The listing builds one solid part. Answer for the finished solid, in the listing's coordinates (mm). A direction names the side the tool comes from. Give positions to 0.01 mm unless a question says otherwise; leave off trailing zeros. Order: outer loops, then holes, each group sorted by start corner. A loop starts at its lowest first (then second) coordinate and runs counter-clockwise, first axis right, second up. Notation, with made-up numbers: (42, -16.5) -> (64, -16.5) arc R21 cw to (64, 0.5) -> close; hole circle Ø6 at (-19, -37.75). An arc over 180 degrees is marked (long way). Answer as a JSON object with one key per item and string values. Group by question number.
```python
from build123d import *

# Parameters (mm, degrees)
F0_W     = 1.2
F0_H     = 0.3
F1_DEPTH = 4.7
F3_DEPTH = 1.05
F6_DEPTH = 2
F7_SIZE  = 1
F8_W     = 2.05
F8_H     = 0.3
F9_DEPTH = 125


with BuildPart() as f1:
    # F0 (on Front) → F1 (new body)
    with BuildSketch(Plane.XZ):
        with BuildLine():
            Line((0, 31.15), (0, 0))
            Line((0, 0), (19.75, 0))
            Line((19.75, 0), (19.75, 31.15))
            Line((19.75, 31.15), (18.55, 31.15))
            Line((18.55, 31.15), (10.275, 31.15))
            Line((10.275, 31.15), (10.275, 31.45))
            Line((10.275, 31.45), (18.55, 31.45))
            Line((18.55, 31.45), (19.75, 31.45))
            Line((19.75, 31.45), (19.75, 52.5))
            Line((19.75, 52.5), (19.75, 55.1716775767))
            ThreePointArc((19.75, 55.1716775767), (18.375, 59.5), (19.75, 63.8283224233))
            Line((19.75, 63.8283224233), (19.75, 65))
            Line((19.75, 65), (0, 65))
            Line((0, 65), (0, 63.8283224233))
            ThreePointArc((0, 63.8283224233), (1.0229892277, 61.7707377656), (1.375, 59.5))
            ThreePointArc((1.375, 59.5), (1.0229892277, 57.2292622344), (0, 55.1716775767))
            Line((0, 55.1716775767), (0, 52.5))
            Line((0, 52.5), (0, 31.45))
            Line((0, 31.45), (1.2, 31.45))
            Line((1.2, 31.45), (9.475, 31.45))
            Line((9.475, 31.45), (9.475, 31.15))
            Line((9.475, 31.15), (1.2, 31.15))
            Line((1.2, 31.15), (0, 31.15))
        make_face()
        with BuildLine():
            Line((-2, 52.5), (0, 52.5))
            Line((0, 52.5), (0, 55.1716775767))
            ThreePointArc((0, 55.1716775767), (-0.9094386331, 54.1103878035), (-2, 53.2362650918))
            Line((-2, 53.2362650918), (-2, 52.5))
        make_face()
        with BuildLine():
            Line((19.75, 55.1716775767), (19.75, 52.5))
            Line((19.75, 52.5), (21.75, 52.5))
            Line((21.75, 52.5), (21.75, 53.2362650918))
            ThreePointArc((21.75, 53.2362650918), (20.6594386331, 54.1103878035), (19.75, 55.1716775767))
        make_face()
        with Locations((0.6, 31.3)):
            Rectangle(F0_W, F0_H)
        with Locations((19.15, 31.3)):
            Rectangle(F0_W, F0_H)
    extrude(amount=F1_DEPTH)

    # F2 (on face) → F3 (cut)
    with BuildSketch(Plane.XZ.offset(4.7)):
        Polygon((13.475, 37.5), (6.275, 37.5), (6.275, 2.2), (6.275, 0), (13.475, 0), (13.475, 2.2), align=None)
    extrude(amount=-F3_DEPTH, mode=Mode.SUBTRACT)

    # F5 (on face) → F6 (join)
    with BuildSketch(Plane.XZ.offset(4.7)):
        with BuildLine():
            Line((-2, 52.5), (0, 52.5))
            Line((0, 52.5), (19.75, 52.5))
            Line((19.75, 52.5), (21.75, 52.5))
            Line((21.75, 52.5), (21.75, 53.2362650918))
            ThreePointArc((21.75, 53.2362650918), (18.5052276407, 58.1084342015), (19.75, 63.8283224233))
            Line((19.75, 63.8283224233), (19.75, 65))
            Line((19.75, 65), (0, 65))
            Line((0, 65), (0, 63.8283224233))
            ThreePointArc((0, 63.8283224233), (1.2447723593, 58.1084342015), (-2, 53.2362650918))
            Line((-2, 53.2362650918), (-2, 52.5))
        make_face()
    extrude(amount=F6_DEPTH)

    # F7
    f7_edges = [f1.edges().sort_by_distance(p)[0] for p in [
        (0, -2.35, 0),
        (19.75, -2.35, 0),
        (3.1375, -4.7, 0),
        (16.6125, -4.7, 0),
        (9.875, -3.65, 0),
    ]]
    chamfer(f7_edges, length=F7_SIZE)

    # F8 (on face) → F9 (cut, symmetric)
    with BuildSketch(Plane(origin=(9.475, 0, 0), x_dir=(0, -1, 0), z_dir=(-1, 0, 0))):
        with Locations((1.825, 31.3)):
            Rectangle(F8_W, F8_H)
    extrude(amount=F9_DEPTH, both=True, mode=Mode.SUBTRACT)


solid = f1.part
```
(1) A cutting plane is placed at B-B (y = -2). Determine the outline of the cut face in (x, z) (3 decimals), and give its area (3 significant figures).
(2) Find the intervals of material crossed by line 1 along Z through (x, y) = (11.75, -0.75); line 2 along X through (y, z) = (-4.5, 5.5) (3 decimals); line 3 along Y through (x, z) = (14.25, 6), in increasing order. Write a range as [from, to].
(3) Flat-ended cylindrical pins translate along their axes: pin 1 Ø8 at (x, z) = (1.5, 31.5) entering from -Y; pin 2 Ø0.8 at (y, z) = (-4, 34) entering from -X; pin 3 Ø3 at (x, y) = (15.5, -5.5) entering from -Z. Find the tip coordinate at first contact, or state that the pin passes through.
(4) For a pull along Z with two mould halves and no side action, classify faces 6 (the flat face through (10, -2, 31.45)), 7 (the flat face through (19.75, -2, 26)), 8 (the flat face through (10, -2, 0)) as +Z half, -Z half, draft (parallel to the pull), parting line (faces both ways), or undercut.
(5) A cutting plane is placed at C-C (z = 34). Determine the outline of the cut face in (x, y) (3 decimals), and give its area (3 significant figures).
(6) A cutting plane is placed at D-D (z = 46). Determine the outline of the cut face in (x, y), and give its area (3 significant figures).
(7) A cutting plane is placed at A-A (x = 5). Determine the outline of the cut face in (y, z), and give its area (3 significant figures).
(8) Which of the six approach directions +Z, -Z, +X, -X, +Y, -Y give full straight-line access (tool end or side, diameter ignored) to faces 1 (the flat face through (0, -2, 27)), 2 (the flat face through (14, -4.7, 27)), 3 (the flat face through (0, -3, 64)), 4 (the flat face through (13.475, -4, 15)), 5 (the flat face through (19.75, -3, 64))?
Check sheet entries:
{
 "1": {"outline": "(-2, 52.5) -> (0, 52.5) -> (0, 31.45) -> (19.75, 31.45) -> (19.75, 52.5) -> (21.75, 52.5) -> (21.75, 53.236) arc R7.5 cw to (19.75, 63.828) -> (19.75, 65) -> (0, 65) -> (0, 63.828) arc R7.5 cw to (-2, 53.236) -> close; (0, 1) -> (1, 0) -> (18.75, 0) -> (19.75, 1) -> (19.75, 31.15) -> (0, 31.15) -> close", "area": "1,270 mm2"},
 "2": {"line 1": "z = [0, 31.15], [31.45, 65]", "line 2": "x = [0, 6.275], [13.475, 19.75]", "line 3": "y = [-4.7, 0]"},
 "3": {"pin 1": "stops at y = -4.7", "pin 2": "stops at x = 0", "pin 3": "stops at z = 0.3"},
 "4": {"face 6": "undercut", "face 7": "draft", "face 8": "-Z half"},
 "5": {"outline": "(0, -4.7) -> (6.275, -4.7) -> (6.275, -3.65) -> (13.475, -3.65) -> (13.475, -4.7) -> (19.75, -4.7) -> (19.75, 0) -> (0, 0) -> close", "area": "85.3 mm2"},
 "6": {"outline": "(0, -4.7) -> (19.75, -4.7) -> (19.75, 0) -> (0, 0) -> close", "area": "92.8 mm2"},
 "7": {"outline": "(-6.7, 52.5) -> (-4.7, 52.5) -> (-4.7, 31.45) -> (0, 31.45) -> (0, 65) -> (-6.7, 65) -> close; (-4.7, 1) -> (-3.7, 0) -> (0, 0) -> (0, 31.15) -> (-4.7, 31.15) -> close", "area": "329 mm2"},
 "8": {"face 1": "-Z, -X, +Y, -Y", "face 2": "-Z, +X, -X, -Y", "face 3": "+Z, -X, +Y, -Y", "face 4": "-Z, -Y", "face 5": "+Z, +X, +Y, -Y"}
}
